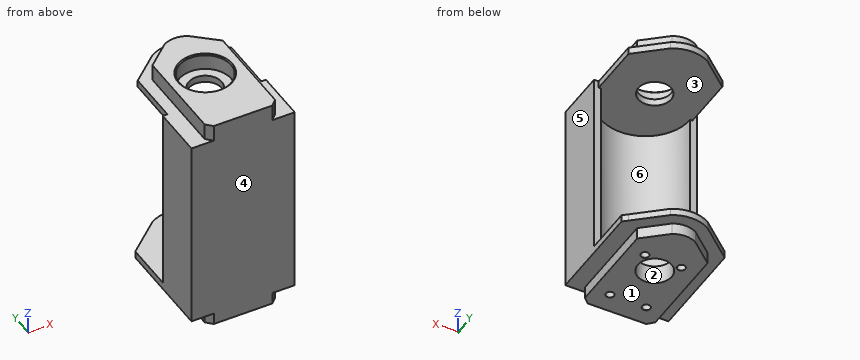
from build123d import *

# Parameters (mm, degrees)
SKETCH3_R                      = 7.25
BOSS_EXTRUDE1_DEPTH            = 5
BOSS_EXTRUDE2_DEPTH            = 80
BOSS_EXTRUDE3_DEPTH            = 10
SKETCH16_R                     = 11
CUT_EXTRUDE1_DEPTH             = 7
CUT_EXTRUDE2_REACH             = 97.699
SKETCH17_R                     = 7
CHAMFER2_SIZE                  = 0.5
CHAMFER3_SIZE                  = 0.5
BOSS_EXTRUDE7_DEPTH            = 3
CUT_EXTRUDE7_DEPTH             = 7
SKETCH3_6_R                    = 7.25
CUT_EXTRUDE6_DEPTH             = 5
BOSS_EXTRUDE8_START            = -5
BOSS_EXTRUDE8_OUTLINE_R        = 7.25
BOSS_EXTRUDE8_DEPTH            = 5
SKETCH24_R                     = 7.25
BOSS_EXTRUDE12_DEPTH           = 3
M3_CLEARANCE_HOLE1_D           = 3.4
M3_CLEARANCE_HOLE1_DEPTH       = 10
M3_CLEARANCE_HOLE1_CSINK_D     = 3.45
M3_CLEARANCE_HOLE1_CSINK_ANGLE = 90
M3_CLEARANCE_HOLE1_TIP         = 1.021463052
CUT_EXTRUDE8_DEPTH             = 5


# Read off the part's stored shape, not the designer's step: Boss-Extrude8
with BuildPart() as part:
    # Sketch3 → Boss-Extrude1 (new body)
    with BuildSketch(Plane.XY):
        with BuildLine():
            Line((22, 0), (22, -22))
            Line((22, -22), (-22, -22))
            Line((-22, -22), (-22, 0))
            ThreePointArc((-22, 0), (0, 22), (22, 0))
        make_face()
        with Locations((0, 7)):
            Circle(SKETCH3_R, mode=Mode.SUBTRACT)
    extrude(amount=BOSS_EXTRUDE1_DEPTH)

    # Sketch7 → Boss-Extrude2 (add)
    with BuildSketch(Plane.XY.offset(5)):
        with BuildLine():
            Line((-19, 0), (-22, 0))
            Line((-22, 0), (-22, -22))
            Line((-22, -22), (22, -22))
            Line((22, -22), (22, 0))
            Line((22, 0), (19, 0))
            ThreePointArc((19, 0), (0, -19), (-19, 0))
        make_face()
    extrude(amount=BOSS_EXTRUDE2_DEPTH)

    # Sketch9 → Boss-Extrude3 (add)
    with BuildSketch(Plane.XY.offset(85)):
        with BuildLine():
            Line((-15, 20.5), (-15, -22))
            Line((-15, -22), (15, -22))
            Line((15, -22), (15, 20.5))
            Line((15, 20.5), (5, 29.160254038))
            ThreePointArc((5, 29.160254038), (0, 30.5), (-5, 29.160254038))
            Line((-5, 29.160254038), (-15, 20.5))
        make_face()
    extrude(amount=BOSS_EXTRUDE3_DEPTH)

    # Sketch16 → Cut-Extrude1 (cut)
    with BuildSketch(Plane.XY.offset(95)):
        with Locations((0, 7)):
            Circle(SKETCH16_R)
    extrude(amount=-CUT_EXTRUDE1_DEPTH, mode=Mode.SUBTRACT)

    # Sketch17 → Cut-Extrude2 (cut, up to next)
    with BuildSketch(Plane.XY.offset(88), mode=Mode.PRIVATE) as cut_extrude2_sk1:
        with Locations((0, 7)):
            Circle(SKETCH17_R)
    cut_extrude2_tool1 = extrude(cut_extrude2_sk1.sketch, amount=-CUT_EXTRUDE2_REACH, mode=Mode.PRIVATE) & part.part
    add(cut_extrude2_tool1.solids().sort_by_distance((0, 7, 88))[0], mode=Mode.SUBTRACT)

    # Chamfer2
    chamfer2_edges = [part.edges().sort_by_distance(p)[0] for p in [
        (-11, 7, 95),
    ]]
    chamfer(chamfer2_edges, length=CHAMFER2_SIZE)

    # Chamfer3
    chamfer3_edges = [part.edges().sort_by_distance(p)[0] for p in [
        (-7.25, 7, 5),
    ]]
    chamfer(chamfer3_edges, length=CHAMFER3_SIZE)

    # Sketch22 → Boss-Extrude7 (add)
    with BuildSketch(Plane(origin=(0, 0, 85), x_dir=(-1, 0, 0), z_dir=(0, 0, -1))):
        with BuildLine():
            Line((-20, 22.784251259), (-20, 0))
            Line((-20, 0), (-20, -11.66190379))
            Line((-20, -11.66190379), (-20, -22))
            Line((-20, -22), (-15, -22))
            Line((-15, -22), (-15, -11.66190379))
            Line((-15, -11.66190379), (-15, 20.5))
            Line((-15, 20.5), (-5, 29.160254038))
            ThreePointArc((-5, 29.160254038), (0, 30.5), (5, 29.160254038))
            Line((5, 29.160254038), (15, 20.5))
            Line((15, 20.5), (15, -11.66190379))
            Line((15, -11.66190379), (15, -22))
            Line((15, -22), (20, -22))
            Line((20, -22), (20, -11.66190379))
            Line((20, -11.66190379), (20, 0))
            Line((20, 0), (20, 22.784251259))
            Line((20, 22.784251259), (7.949555075, 33.220242691))
            ThreePointArc((7.949555075, 33.220242691), (0, 35.5), (-7.949555075, 33.220242691))
            Line((-7.949555075, 33.220242691), (-20, 22.784251259))
        make_face()
        Polygon((22, 0), (20, 0), (20, -11.66190379), (20, -22), (22, -22), align=None)
        Polygon((-20, -11.66190379), (-20, 0), (-22, 0), (-22, -22), (-20, -22), align=None)
    extrude(amount=-BOSS_EXTRUDE7_DEPTH)

    # Sketch25 → Cut-Extrude7 (cut)
    with BuildSketch(Plane.XY.offset(95)):
        Polygon((-15, -19.5), (-12.5, -22), (-15, -22), align=None)
        Polygon((15, -19.5), (12.5, -22), (15, -22), align=None)
    extrude(amount=-CUT_EXTRUDE7_DEPTH, mode=Mode.SUBTRACT)

    # Sketch3<6> → Cut-Extrude6 (cut)
    # profile 1 of 3: a face of its own
    with BuildSketch(Plane.XY):
        with BuildLine():
            ThreePointArc((0, -22), (15.556349186, -15.556349186), (22, 0))
            ThreePointArc((22, 0), (0, 22), (-22, 0))
            ThreePointArc((-22, 0), (-15.556349186, -15.556349186), (0, -22))
        make_face()
        with Locations((0, 7)):
            Circle(SKETCH3_6_R, mode=Mode.SUBTRACT)
    # profile 2 of 3: a face of its own
    with BuildSketch(Plane.XY):
        with BuildLine():
            ThreePointArc((0, -22), (-15.556349186, -15.556349186), (-22, 0))
            Line((-22, 0), (-22, -22))
            Line((-22, -22), (0, -22))
        make_face()
    # profile 3 of 3: a face of its own
    with BuildSketch(Plane.XY):
        with BuildLine():
            Line((22, -22), (22, 0))
            ThreePointArc((22, 0), (15.556349186, -15.556349186), (0, -22))
            Line((0, -22), (22, -22))
        make_face()
    extrude(amount=CUT_EXTRUDE6_DEPTH, mode=Mode.SUBTRACT)

    # Boss-Extrude8 outline → Boss-Extrude8 (add)
    with BuildSketch(Plane(origin=(0, 0, 0), x_dir=(-1, 0, 0), z_dir=(0, 0, -1)).offset(BOSS_EXTRUDE8_START)):
        with BuildLine():
            Line((15, 20.5), (5, 29.160254038))
            ThreePointArc((5, 29.160254038), (0, 30.5), (-5, 29.160254038))
            Line((-5, 29.160254038), (-15, 20.5))
            Line((-15, 20.5), (-15, -22))
            Line((-15, -22), (15, -22))
            Line((15, -22), (15, 20.5))
        make_face()
        with Locations((0, 7)):
            Circle(BOSS_EXTRUDE8_OUTLINE_R, mode=Mode.SUBTRACT)
    extrude(amount=BOSS_EXTRUDE8_DEPTH)

    # Sketch24 → Boss-Extrude12 (add)
    with BuildSketch(Plane(origin=(0, 0, 5), x_dir=(-1, 0, 0), z_dir=(0, 0, -1))):
        with BuildLine():
            Line((-7.949555075, 33.220242691), (-20, 22.784251259))
            Line((-20, 22.784251259), (-22, 21.052200451))
            Line((-22, 21.052200451), (-22, 0))
            Line((-22, 0), (-22, -22))
            Line((-22, -22), (22, -22))
            Line((22, -22), (22, 0))
            Line((22, 0), (22, 21.052200451))
            Line((22, 21.052200451), (20, 22.784251259))
            Line((20, 22.784251259), (7.949555075, 33.220242691))
            ThreePointArc((7.949555075, 33.220242691), (0, 35.5), (-7.949555075, 33.220242691))
        make_face()
        with Locations((0, 7)):
            Circle(SKETCH24_R, mode=Mode.SUBTRACT)
    extrude(amount=-BOSS_EXTRUDE12_DEPTH)

    # M3 Clearance Hole1
    with Locations(Plane(origin=(0, 0, 0), x_dir=(-1, 0, 0), z_dir=(0, 0, -1))):
        with Locations((7.75, 13.423393759), (-7.75, 13.423393759), (-7.75, -13.423393759), (7.75, -13.423393759)):
            CounterSinkHole(M3_CLEARANCE_HOLE1_D / 2, M3_CLEARANCE_HOLE1_CSINK_D / 2, depth=M3_CLEARANCE_HOLE1_DEPTH, counter_sink_angle=M3_CLEARANCE_HOLE1_CSINK_ANGLE)
            with Locations((0, 0, -(M3_CLEARANCE_HOLE1_DEPTH + M3_CLEARANCE_HOLE1_TIP / 2))):  # 118° drill point
                Cone(0, M3_CLEARANCE_HOLE1_D / 2, M3_CLEARANCE_HOLE1_TIP, mode=Mode.SUBTRACT)

    # Sketch26 → Cut-Extrude8 (cut)
    with BuildSketch(Plane(origin=(0, 0, 0), x_dir=(-1, 0, 0), z_dir=(0, 0, -1))):
        Polygon((-15, -19.5), (-12.5, -22), (-15, -22), align=None)
        Polygon((15, -19.5), (12.5, -22), (15, -22), align=None)
    extrude(amount=-CUT_EXTRUDE8_DEPTH, mode=Mode.SUBTRACT)


solid = part.part
The listing builds one solid part. Answer for the finished solid, in the listing's coordinates (mm). Face numbers are marked on the shaded views. A direction names the side the tool comes from. Coordinates: 2 decimals unless noted, no trailing zeros. Order: outer loops, then holes, each group sorted by start corner. A loop starts at its lowest first (then second) coordinate and runs counter-clockwise, first axis right, second up.
Q1. A cutting plane is placed at C-C, the plane z = 29. Write down the section's boundary in (x, y).
Q2. Given P1, Ø2.5, axis at x = 7.75, y = 13.42, coming from the +Z side; P2, Ø1.5, axis at x = 21, z = 60.5, coming from the +Y side; P3, Ø3.5, axis at y = 11.5, z = 86.5, coming from the -X side, each flat-ended and moving along its own axis, determine where each tip first touches the part or whether it passes through.
Q3. For a pull along X with two mould halves and no side action, classify the marked faces 4, 5 and 6 as pulls with the +X half, pulls with the -X half, needs draft (parallel to the pull), parting line crosses it, or undercut.
Q4. A cutting plane is placed at D-D, the plane x = 18. Write down the section's boundary in (y, z).
Q5. A cutting plane is placed at A-A, the plane y = 7. State how many separate pieces and enclosed holes the cut face has, and give its area (3 significant figures).
Q6. A cutting plane is placed at B-B, the plane x = 0. Write down the section's boundary in (y, z).
Q7. Consider line 1 (Z direction, x = -15.5, y = 22); line 2 (Z direction, x = -2, y = 22); line 3 (Y direction, x = 0, z = 86). Determine where each line is inside the solid, lowest interval first.
Q8. Which of the six approach directions +Z, -Z, +X, -X, +Y, -Y give full straight-line access (tool end or side, diameter ignored) to the marked faces 1, 2 and 3?
Answers follow:
1. outline: (-22, -22) - (22, -22) - (22, 0) - (19, 0) arc R19 cw to (-19, 0) - (-22, 0) - close
2. P1: stops at z = 94.81
2. P2: stops at y = 0
2. P3: stops at x = -20
3. face 4: needs draft
3. face 5: pulls with the +X half
3. face 6: undercut
4. outline: (-22, 5) - (24.52, 5) - (24.52, 8) - (-6.08, 8) - (-6.08, 85) - (24.52, 85) - (24.52, 88) - (-22, 88) - close
5. separate pieces: 4
5. enclosed holes: 0
5. area: 300 mm2
6. outline: (-22, 0) - (-0.25, 0) - (-0.25, 8) - (-19, 8) - (-19, 85) - (0, 85) - (0, 88) - (-4, 88) - (-4, 94.5) - (-4.5, 95) - (-22, 95) - close; (14, 85) - (35.5, 85) - (35.5, 88) - (30.5, 88) - (30.5, 95) - (18.5, 95) - (18, 94.5) - (18, 88) - (14, 88) - close; (14.25, 0) - (30.5, 0) - (30.5, 5) - (35.5, 5) - (35.5, 8) - (14.25, 8) - close
7. line 1: z = 5 to 8, 85 to 88
7. line 2: z = 0 to 8, 85 to 95
7. line 3: y = -22 to 0, 14 to 35.5
8. face 1: -Z, +X, -X, +Y, -Y
8. face 2: -Z
8. face 3: +Y
